CAD build for the part. Positions are in the model's coordinates, mm. Face numbers are marked on the shaded views. A direction names the side the tool comes from. Round coordinates to 2 decimals unless told otherwise and drop trailing zeros. Order: outer loops, then holes, each group sorted by start corner. A loop starts at its lowest first (then second) coordinate and runs counter-clockwise, first axis right, second up. Notation, with made-up numbers: (50, 35) - (78, 35) arc R5 cw to (78, 41) - close; hole circle Ø4 at (-22, 77.25). An arc over 180 degrees is marked (long way). Write item = value, one per line.
from build123d import *

# Parameters (mm, degrees)
F0_W     = 22.86
F0_H     = 50.8
F1_DEPTH = 50.8


with BuildPart() as f1:
    # F0 (on Top) → F1 (new body)
    with BuildSketch(Plane.XY):
        Polygon((56.896489, 42.170627), (-6.603511, 42.170627), (-70.103511, 42.170627), (-70.103511, 32.525493), (-61.213511, 32.525493), (-61.213511, -22.084507), (-70.103511, -22.084507), (-70.103511, -28.949373), (56.896489, -28.949373), (56.896489, -22.084507), (48.006489, -22.084507), (48.006489, 32.525493), (56.896489, 32.525493), align=None)
        with Locations((-37.083511, 4.070627)):
            Rectangle(F0_W, F0_H, mode=Mode.SUBTRACT)
        with Locations((-6.603511, 4.070627)):
            Rectangle(F0_W, F0_H, mode=Mode.SUBTRACT)
        with Locations((23.876489, 4.070627)):
            Rectangle(F0_W, F0_H, mode=Mode.SUBTRACT)
    extrude(amount=F1_DEPTH)


solid = f1.part
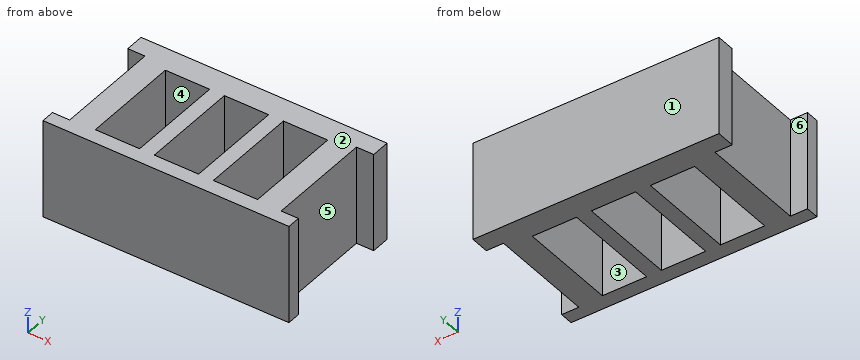
(1) Tool access for the marked faces 4, 5 and 6: list every direction of +Z, -Z, +X, -X, +Y, -Y with a clear straight run to the whole face (end or side of a thin tool).
Solved:
face_4 = +Z, -Z
face_5 = +Z, -Z, +X
face_6 = +Z, -Z, -X
(2) Pull direction Y, two halves, no side cores. Call the marked faces 1, 2 and 3: released by +Y, released by -Y, zero draft, split by the parting line, or undercut.
Solved:
face_1 = released by +Y
face_2 = zero draft
face_3 = undercut
(3) Drop flat-ended pins along their axis: pin 1 (12 mm diameter, centred on x = -19, y = -12, fed in from -Z); pin 2 (15 mm diameter, centred on y = 3, z = 31.5, fed in from -X); pin 3 (15 mm diameter, centred on y = 4.5, z = 17, fed in from +X). Give the stop position or say it passes through.
Solved:
pin_1 = 0
pin_2 = -61.21
pin_3 = 48.01
(4) Band-saw the part on A-A on x = 22. List the corners of the cut face in (y, z), plus the area to 3 significant figures.
Solved:
outline = (-28.95, 0) - (-21.33, 0) - (-21.33, 50.8) - (-28.95, 50.8) - close; (29.47, 0) - (42.17, 0) - (42.17, 50.8) - (29.47, 50.8) - close
area = 1,030 mm²
(5) Probe line 1 along X through (y, z) = (16, 13.5); line 2 along Y through (x, z) = (-14.5, 21.5); line 3 along Y through (x, z) = (51.5, 42.5). List the from-to ranges inside material, lowest first.
Solved:
line_1 = -61.21 to -48.51, -25.65 to -18.03, 4.83 to 12.45, 35.31 to 48.01
line_2 = -28.95 to -21.33, 29.47 to 42.17
line_3 = -28.95 to -22.08, 32.53 to 42.17
(6) Band-saw the part on C-C on z = 46.5. List the corners of the cut face in (x, y), plus the area to 3 significant figures.
Solved:
outline = (-70.1, -28.95) - (56.9, -28.95) - (56.9, -22.08) - (48.01, -22.08) - (48.01, 32.53) - (56.9, 32.53) - (56.9, 42.17) - (-70.1, 42.17) - (-70.1, 32.53) - (-61.21, 32.53) - (-61.21, -22.08) - (-70.1, -22.08) - close; hole (-48.51, -21.33) - (-25.65, -21.33) - (-25.65, 29.47) - (-48.51, 29.47) - close; hole (-18.03, -21.33) - (4.83, -21.33) - (4.83, 29.47) - (-18.03, 29.47) - close; hole (12.45, -21.33) - (35.31, -21.33) - (35.31, 29.47) - (12.45, 29.47) - close
area = 4,580 mm²
(7) Band-saw the part on B-B on y = -11. List the corners of the cut face in (x, z), plus the area to 3 significant figures.
Solved:
outline = (-61.21, 0) - (-48.51, 0) - (-48.51, 50.8) - (-61.21, 50.8) - close; (-25.65, 0) - (-18.03, 0) - (-18.03, 50.8) - (-25.65, 50.8) - close; (4.83, 0) - (12.45, 0) - (12.45, 50.8) - (4.83, 50.8) - close; (35.31, 0) - (48.01, 0) - (48.01, 50.8) - (35.31, 50.8) - close
area = 2,060 mm²
